Autodesk Inventor part; units mm, degrees
ref_plane "YZ Plane" through (0, 0, 0) normal (1, 0, 0) x (0, 1, 0)
ref_plane "XZ Plane" through (0, 0, 0) normal (0, 1, 0) x (-1, 0, 0)
ref_plane "XY Plane" through (0, 0, 0) normal (0, 0, 1) x (1, 0, 0)
sketch "Sketch1" plane through (0, 0, 0) normal (0, 0, 1) x (1, 0, 0)
  circle A0 centre (0, 0) radius 6.1
  line L0 (-6.1, 0) -> (-6.1, -6.1)
  line L1 (-6.1, -6.1) -> (6.1, -6.1)
  line L2 (6.1, -6.1) -> (6.1, 0)
  dimension "d0" = 12.2
extrude "Extrusion1" add sketch "Sketch1" along normal blind 19.05
sketch "Sketch2" plane through (0, 0, 19.05) normal (0, 0, 1) x (1, 0, 0)
  arc A0 (6.1, 0) -> (-6.1, 0) centre (0, 0) ccw construction
  line L0 (-6.1, 0) -> (-6.1, -6.1) construction
  line L1 (6.1, -6.1) -> (6.1, 0) construction
  line L2 (-6.1, -6.1) -> (-6.1, 6.1)
  line L3 (-6.1, 6.1) -> (6.1, 6.1)
  line L4 (6.1, 6.1) -> (6.1, -6.1)
  line L5 (-6.1, -6.1) -> (6.1, -6.1)
extrude "Extrusion2" add sketch "Sketch2" along normal blind 17.78
sketch "Sketch3" plane through (0, 6.1, 19.05) normal (0, 1, 0) x (1, 0, 0)
  line L0 (0, 0) -> (-6.1, 0) construction
  line L1 (-12.6, -8.79) -> (12.6, -8.79) construction
  line L2 (-12.6, -15.04) -> (12.6, -15.04)
  line L3 (12.6, -2.54) -> (-12.6, -2.54)
  arc A0 (-12.6, -2.54) -> (-12.6, -15.04) centre (-12.6, -8.79) ccw
  arc A1 (12.6, -15.04) -> (12.6, -2.54) centre (12.6, -8.79) ccw
  point P0 (0, 19.05)
  point P1 (0, -8.79)
  point P2 (0, -2.54)
  dimension "d5" = 2.54
  dimension "d6" = 25.2
  dimension "d7" = 12.5
extrude "Extrusion3" add sketch "Sketch3" along normal blind 27.25
sketch "Sketch4" plane through (0, 6.1, 19.05) normal (0, -1, 0) x (1, 0, 0)
  arc A0 (12.6, 2.54) -> (12.6, 15.04) centre (12.6, 8.79) ccw construction
  line L0 (-18.85, 0) -> (18.85, 0)
  line L1 (18.85, 0) -> (18.85, 17.78)
  line L2 (18.85, 17.78) -> (-18.85, 17.78)
  line L3 (-18.85, 17.78) -> (-18.85, 0)
  arc A1 (-12.6, 15.04) -> (-12.6, 2.54) centre (-12.6, 8.79) ccw construction
  line L4 (-6.1, 17.78) -> (6.1, 17.78) construction
  point P0 (0, -19.05)
  point P1 (-18.85, 8.79)
  point P2 (18.85, 8.79)
  point P3 (0, 17.78)
  point P4 (0, 0)
extrude "Extrusion4" add sketch "Sketch4" against normal blind 17.25
sketch "Sketch5" plane through (0, 6.1, 19.05) normal (0, -1, 0) x (1, 0, 0)
  line L0 (-18.85, 0) -> (-6.1, 0) construction
  line L1 (18.85, 17.78) -> (-18.85, 17.78)
  line L2 (-18.85, 17.78) -> (-18.85, 0)
  line L3 (-18.85, 0) -> (18.85, 0)
  line L4 (18.85, 0) -> (18.85, 17.78)
  point P0 (0, -19.05)
extrude "Extrusion5" add sketch "Sketch5" along normal up to surface (12.2 mm away)
chamfer "Chamfer1" distance 3.175 angle 45 4 edges at (18.85, 8.625, 19.05) (18.85, 8.625, 36.83) (-18.85, 8.625, 19.05) (-18.85, 8.625, 36.83)
sketch "Sketch6" plane through (-6.1, -6.1, 0) normal (0, -1, 0) x (1, 0, 0)
  line L0 (0, 0) -> (12.2, 0) construction
  line L1 (24.95, 33.655) -> (24.95, 22.225) construction
  line L2 (-9.575, 36.83) -> (21.775, 36.83) construction
  line L3 (21.3, 12.9) -> (21.3, 0.2)
  line L4 (24.95, 27.84) -> (24.95, 22.225) construction
  line L5 (24.95, 22.225) -> (21.775, 22.225)
  line L6 (21.775, 22.225) -> (21.3, 12.9)
  line L7 (24.95, 22.225) -> (24.95, 33.655)
  line L8 (24.95, 33.655) -> (27.49, 33.655)
  line L9 (27.49, 33.655) -> (28.92, 12.9)
  line L10 (28.92, 12.9) -> (28.92, 0.2)
  line L11 (28.92, 0.2) -> (21.3, 0.2)
  line L12 (6.1, 0) -> (6.1, 36.83)
  line L13 (-12.75, 22.225) -> (-9.575, 19.05) construction
  line L14 (-12.75, 33.655) -> (-12.75, 22.225) construction
  line L15 (-9.1, 12.9) -> (-9.1, 0.2)
  line L16 (-12.75, 27.84) -> (-12.75, 22.225) construction
  line L17 (-12.75, 22.225) -> (-9.575, 22.225)
  line L18 (-9.575, 22.225) -> (-9.1, 12.9)
  line L19 (-12.75, 22.225) -> (-12.75, 33.655)
  line L20 (-12.75, 33.655) -> (-15.29, 33.655)
  line L21 (-15.29, 33.655) -> (-16.72, 12.9)
  line L22 (-16.72, 12.9) -> (-16.72, 0.2)
  line L23 (-16.72, 0.2) -> (-9.1, 0.2)
  point P0 (6.1, 0)
  dimension "d17" = 15.2
  dimension "d19" = 0.2
  dimension "d21" = 7.62
  dimension "d23" = 12.7
  dimension "d28" = 2.54
  dimension "d29" = 3.175
extrude "Extrusion6" add sketch "Sketch6" against normal blind 14
fillet "Fillet1" radius 3.175 6 edges at (21.39, 0.9, 33.655) (-21.39, 0.9, 33.655) (-22.82, 0.9, 0.2) (-22.82, 0.9, 12.9) (22.82, 0.9, 0.2) (22.82, 0.9, 12.9)
properties part number "SecondarySecure"
Geometry: final body of the model. Coordinates: model frame, mm. A direction names the side the tool comes from. Give positions to 0.01 mm unless a question says otherwise; leave off trailing zeros. Loops run counter-clockwise (first coordinate to the right, second up) from the corner with the lowest first, then second, coordinate; pieces in that order, holes last. Notation, with made-up numbers: (24, 29) - (77, 29) arc R27 ccw to (77, 46) - close; hole circle Ø9 at (-10, 59.5). An arc over 180 degrees is marked (long way). Answer as CSV lines item,"result". Start each with the question number.
1. Section C-C, the plane x = 0. Return loops of the section in (y, z).
2. Draft query along Z for faces 4 (the face through (17.24, 15.733, 20.615)), 5 (the face through (15.2, 1, 7)), 6 (the face through (18.85, 28.28, 27.7)), 7 (the face through (-15.36, 0.8, 16.02)). Return one class per face: released by +Z, released by -Z, zero draft, split by the parting line, or undercut.
3. Ray query, L1, parallel to X at y = -4, z = 10.5; L2, parallel to Z at x = -3, y = 7; L3, parallel to X at y = 22, z = 30.5. Return the intervals inside material, ascending.
4. Pin query (flat end, axial travel): P1, Ø9, axis at y = 18.5, z = 30.5, coming from the +X side; P2, Ø5, axis at x = -16.5, y = -0.5, coming from the -Z side; P3, Ø4, axis at x = 18, y = 23.5, coming from the -Z side. Return the tip coordinate at first contact, or that it passes through.
5. Reachability of faces 1 (the face through (0, 28, 21.59)), 2 (the face through (-17, 1, 0.2)), 3 (the face through (-0.1, 6.1, 9.4)) from +Z, -Z, +X, -X, +Y, -Y: full face, straight path, thin tool, end or side. Return the list, or none.
6. Section A-A, the plane z = 5. Return loops of the section in (x, y).
7. Section B-B, the plane y = 11.5. Return loops of the section in (x, z) (3 decimals).
8. Section D-D, the plane z = 33. Return loops of the section in (x, y).
Answers:
1,outline,"(-6.1, 0) - (6.1, 0) - (6.1, 19.05) - (23.35, 19.05) - (23.35, 21.59) - (33.35, 21.59) - (33.35, 34.09) - (23.35, 34.09) - (23.35, 36.83) - (-6.1, 36.83) - close"
2,face 4,"released by -Z"
2,face 5,"zero draft"
2,face 6,"split by the parting line"
2,face 7,"undercut"
3,L1,"x = -22.82 to -15.2, -6.1 to 6.1, 15.2 to 22.82"
3,L2,"z = 19.05 to 36.83"
3,L3,"x = -18.85 to 18.85"
4,P1,"stops at x = 18.85"
4,P2,"stops at z = 0.2"
4,P3,"stops at z = 19.38"
5,face 1,"-Z, +X, -X, +Y"
5,face 2,"-Z, -X, +Y, -Y"
5,face 3,"-Z, +Y"
6,outline,"(-22.82, -6.1) - (-15.2, -6.1) - (-15.2, 7.9) - (-22.82, 7.9) - close; (-6.1, -6.1) - (6.1, -6.1) - (6.1, 0) arc R6.1 ccw to (-6.1, 0) - close; (15.2, -6.1) - (22.82, -6.1) - (22.82, 7.9) - (15.2, 7.9) - close"
7,outline,"(-18.85, 22.225) - (-15.675, 19.05) - (15.675, 19.05) - (18.85, 22.225) - (18.85, 33.655) - (15.675, 36.83) - (-15.675, 36.83) - (-18.85, 33.655) - close"
8,outline,"(-20.39, -6.1) - (20.39, -6.1) - (20.39, 7.9) - (18.85, 7.9) - (18.85, 23.35) - (16.13, 23.35) - (16.13, 33.35) - (-16.13, 33.35) - (-16.13, 23.35) - (-18.85, 23.35) - (-18.85, 7.9) - (-20.39, 7.9) - close"
